```python
from build123d import *

# Parameters (mm, degrees)
F3_DEPTH      = 50.8
F3_DEPTH_BACK = 50.8


with BuildPart() as f1:
    # F0 (on Front) → F1 (revolve)
    with BuildSketch(Plane.XZ):
        Polygon((-24.5717495672, 15.875), (-24.5717495672, 6.35), (26.2282504328, 6.35), (26.2282504328, 15.875), (13.5282504328, 19.05), (-11.8717495672, 19.05), align=None)
    revolve(axis=Axis((0.4141309397, 0, 0), (1, 0, 0)))

    # F2 (on Right) → F3 (cut, two sides)
    with BuildSketch(Plane.YZ) as f3_sk:
        Polygon((7.2894281006, 0.7921939781), (2.9586539406, 6.7089269033), (-4.3307741601, 5.9167329252), (-7.2894281006, -0.7921939781), (-2.9586539406, -6.7089269033), (4.3307741601, -5.9167329252), align=None)
    extrude(amount=-F3_DEPTH, mode=Mode.SUBTRACT)
    extrude(f3_sk.sketch, amount=F3_DEPTH_BACK, mode=Mode.SUBTRACT)


solid = f1.part
```
For this review, take the finished solid that the model builds, in its own axes (mm). A direction names the side the tool comes from. Round coordinates to 2 decimals unless told otherwise and drop trailing zeros. Write each loop counter-clockwise with the first axis right and the second up, starting at its lowest first coordinate (ties: lowest second). Pieces come first, ordered by that corner, then holes. Notation, with made-up numbers: (23.5, 4.5) - (46.5, 4.5) arc R12 cw to (46.5, 20.5) - close; hole circle Ø6 at (49.25, -16.75). An arc over 180 degrees is marked (long way). Use CSV: the item, a comma, the result in double quotes.
1) Add section D-D on x = 15.5. Write out the cut boundary in (y, z), and give its area (3 significant figures).
Conclusion:
outline,"circle Ø37.11 at (0, 0); hole (-7.29, -0.79) - (-2.96, -6.71) - (4.33, -5.92) - (7.29, 0.79) - (2.96, 6.71) - (-4.33, 5.92) - close"
area,"942 mm^2"
2) Add section A-A on y = 0. Write out the cut boundary in (x, z) (3 decimals).
Conclusion:
outline,"(-24.572, -15.875) - (-11.872, -19.05) - (13.528, -19.05) - (26.228, -15.875) - (26.228, -6.387) - (-24.572, -6.387) - close; (-24.572, 6.387) - (26.228, 6.387) - (26.228, 15.875) - (13.528, 19.05) - (-11.872, 19.05) - (-24.572, 15.875) - close"
3) Add section C-C on z = 0. Write out the cut boundary in (x, y) (3 decimals).
Conclusion:
outline,"(-24.572, -15.875) - (-11.872, -19.05) - (13.528, -19.05) - (26.228, -15.875) - (26.228, -6.94) - (-24.572, -6.94) - close; (-24.572, 6.94) - (26.228, 6.94) - (26.228, 15.875) - (13.528, 19.05) - (-11.872, 19.05) - (-24.572, 15.875) - close"
4) The part is to be moulded in two halves that separate along Z. For faces 3 (the cylindrical face through (0.65, 11.59, -15.12)), 4 (the flat face through (26.228, 0, -7)), 5 (the flat face through (1.184, -0.635, 6.318)), 6 (the flat face through (1.18, -5.79, 2.61)), say which applies: pulls with the +Z half, pulls with the -Z half, needs draft (parallel to the pull), parting line crosses it, or undercut.
Conclusion:
face 3,"parting line crosses it"
face 4,"needs draft"
face 5,"undercut"
face 6,"undercut"
5) Add section B-B on x = -2. Write out the cut boundary in (y, z), and give its area (3 significant figures).
Conclusion:
outline,"circle Ø38.1 at (0, 0); hole (-7.29, -0.79) - (-2.96, -6.71) - (4.33, -5.92) - (7.29, 0.79) - (2.96, 6.71) - (-4.33, 5.92) - close"
area,"1,000 mm^2"
6) For faces 1 (the flat face through (1.184, 0.635, -6.318)), 2 (the flat face through (-24.572, 0, 7)), list the 3-axis set-ups (+Z, -Z, +X, -X, +Y, -Y) from which the entire face can be reached by the end or side of a thin tool; tool diameter is ignored.
Conclusion:
face 1,"+X, -X"
face 2,"+Z, -Z, -X, +Y, -Y"
7) Wall thickness on line 1 along Y through (x, z) = (-12.5, -2); line 2 along Z through (x, y) = (1, -2.5); line 3 along Z through (x, y) = (-11, -6.5): over which ranges is each line inside the solid? List them lowest first. Write a range as from..to.
Conclusion:
line 1,"y = -18.79..-6.41, 6.06..18.79"
line 2,"z = -18.89..-6.66, 6.12..18.89"
line 3,"z = -17.91..-1.87, 1..17.91"
8) Clearance check with flat-ended pins moving along their axes: pin 1 Ø3 at (x, y) = (-4.5, -12) entering from -Z; pin 2 Ø5 at (x, y) = (12.5, -7.5) entering from -Z; pin 3 Ø4 at (x, y) = (-1, 5) entering from +Z; pin 4 Ø5 at (x, y) = (-11.5, 1.5) entering from -Z. State where each tip first meets the part, or that it passes through.
Conclusion:
pin 1,"stops at z = -15.9"
pin 2,"stops at z = -18.38"
pin 3,"stops at z = 18.81"
pin 4,"stops at z = -19.05"
